from build123d import *

# Parameters (mm, degrees)
F0_W     = 100
F0_H     = 50
F1_DEPTH = 80
F2_W     = 90
F2_H     = 40
F3_DEPTH = 75
F4_R     = 4.99999
F5_R     = 10
F6_SIZE  = 1
F8_DEPTH = 5


# Not quite as in the source:
# - a fillet or chamfer is up to 0.001 mm smaller than in the source, because OpenCascade refuses the exact size


with BuildPart() as f1:
    # F0 (on Top) → F1 (new body)
    with BuildSketch(Plane.XY):
        Rectangle(F0_W, F0_H)
    extrude(amount=F1_DEPTH)

    # F2 (on face) → F3 (cut)
    with BuildSketch(Plane.XY.offset(80)):
        Rectangle(F2_W, F2_H)
    extrude(amount=-F3_DEPTH, mode=Mode.SUBTRACT)

    # F4 (radius 5 in the source; OpenCascade refuses exactly that, so slightly less here)
    f4_edges = [f1.edges().sort_by_distance(p)[0] for p in [
        (45, 0, 5),
        (0, 20, 5),
        (0, -20, 5),
        (-45, 0, 5),
        (-45, 20, 42.5),
        (-45, -20, 42.5),
        (45, 20, 42.5),
        (45, -20, 42.5),
        (45, 0, 80),
        (0, 20, 80),
        (-45, 0, 80),
        (0, -20, 80),
    ]]
    fillet(f4_edges, radius=F4_R)

    # F5
    f5_edges = [f1.edges().sort_by_distance(p)[0] for p in [
        (50, -25, 40),
        (-50, -25, 40),
        (-50, 25, 40),
        (50, 25, 40),
    ]]
    fillet(f5_edges, radius=F5_R)

    # F6
    f6_edges = [f1.edges().sort_by_distance(p)[0] for p in [
        (0, -25, 0),
        (47.071068, -22.071068, 0),
        (50, 0, 0),
        (47.071068, 22.071068, 0),
        (0, 25, 0),
        (-47.071068, 22.071068, 0),
        (-50, 0, 0),
        (-47.071068, -22.071068, 0),
    ]]
    chamfer(f6_edges, length=F6_SIZE)

    # F7 (on face) → F8 (cut)
    with BuildSketch(Plane.XZ.offset(25)):
        with BuildLine():
            Line((25, 55), (-25, 55))
            ThreePointArc((-25, 55), (-28.5355339059, 53.5355339059), (-30, 50))
            Line((-30, 50), (-30, 31))
            ThreePointArc((-30, 31), (-28.5355339059, 27.4644660941), (-25, 26))
            Line((-25, 26), (25, 26))
            ThreePointArc((25, 26), (28.5355339059, 27.4644660941), (30, 31))
            Line((30, 31), (30, 50))
            ThreePointArc((30, 50), (28.5355339059, 53.5355339059), (25, 55))
        make_face()
    extrude(amount=-F8_DEPTH, mode=Mode.SUBTRACT)


solid = f1.part
Design review of the part built by this model. Coordinates are the model's own, in mm. A direction names the side the tool comes from. Round coordinates to 2 decimals unless told otherwise and drop trailing zeros. Write each loop counter-clockwise with the first axis right and the second up, starting at its lowest first coordinate (ties: lowest second). Pieces come first, ordered by that corner, then holes.
Item 1: For faces 1 (the flat face through (-30, -23, 41)), 2 (the cylindrical face through (-47.15, -21.99, 41.05)), 3 (the cylindrical face through (1, -19, 7)), list the 3-axis set-ups (+Z, -Z, +X, -X, +Y, -Y) from which the entire face can be reached by the end or side of a thin tool; tool diameter is ignored.
Item 2: Consider section D-D on z = 48. Give the boundary of the cut face in (x, y), and give its area (3 significant figures).
Item 3: Wall thickness on L1, parallel to Y at x = -6, z = 22; L2, parallel to X at y = 1, z = 74; L3, parallel to Z at x = -4.5, y = 3.5: over which ranges is each line inside the solid? List them lowest first.
Item 4: Consider section A-A on z = 21.5. Give the boundary of the cut face in (x, y).
Item 5: For pin 1 Ø3 at (x, y) = (6, -1.5) entering from +Z; pin 2 Ø4 at (x, y) = (0, -22) entering from +Z; pin 3 Ø2.5 at (y, z) = (-23, 43) entering from -X, all flat-tipped, find the tip position at first contact; note any pin that passes through.
Item 6: Draft analysis for pull direction Z (two halves, no side actions). For faces 4 (the cylindrical face through (29, -23, 53)), 5 (the cylindrical face through (43, -19, 42)), 6 (the flat face through (-1, 0, 0)), state which applies: released by +Z, released by -Z, zero draft, split by the parting line, or undercut.
Check values:
1. face 1: -Y
1. face 2: +Z, -Z, -X, -Y
1. face 3: +Z
2. outline: (-50, -15) arc R10 ccw to (-40, -25) - (-30, -25) - (-30, -20) - (-40, -20) arc R5 cw to (-45, -15) - (-45, 15) arc R5 cw to (-40, 20) - (40, 20) arc R5 cw to (45, 15) - (45, -15) arc R5 cw to (40, -20) - (30, -20) - (30, -25) - (40, -25) arc R10 ccw to (50, -15) - (50, 15) arc R10 ccw to (40, 25) - (-40, 25) arc R10 ccw to (-50, 15) - close
2. area: 1,040 mm2
3. L1: y = -25 to -20, 20 to 25
3. L2: x = -50 to -45, 45 to 50
3. L3: z = 0 to 5
4. outline: (-50, -15) arc R10 ccw to (-40, -25) - (40, -25) arc R10 ccw to (50, -15) - (50, 15) arc R10 ccw to (40, 25) - (-40, 25) arc R10 ccw to (-50, 15) - close; hole (-45, -15) arc R5 ccw to (-40, -20) - (40, -20) arc R5 ccw to (45, -15) - (45, 15) arc R5 ccw to (40, 20) - (-40, 20) arc R5 ccw to (-45, 15) - close
5. pin 1: stops at z = 5
5. pin 2: stops at z = 79.9
5. pin 3: stops at x = -47.38
6. face 4: undercut
6. face 5: zero draft
6. face 6: released by -Z
